```python
from build123d import *

# Parameters (mm, degrees)
SKETCH1_W           = 55
SKETCH1_H           = 4
SKETCH1_W_2         = 4.6
SKETCH1_H_2         = 5
BOSS_EXTRUDE2_DEPTH = 30
FILLET1_R           = 1
SKETCH2_R           = 2.5
SKETCH2_W           = 6.2
SKETCH2_H           = 6.2
CUT_EXTRUDE1_DEPTH  = 10
SKETCH4_W           = 19.295263263
SKETCH4_H           = 1.550295644
SKETCH4_W_2         = 7.637827672
SKETCH4_H_2         = 1.509017847
SKETCH4_W_3         = 7.600819518
SKETCH4_H_3         = 1.495167717
CUT_EXTRUDE2_DEPTH  = 25


with BuildPart() as part:
    # Sketch1 → Boss-Extrude2 (new body)
    with BuildSketch(Plane.XY):
        Rectangle(SKETCH1_W, SKETCH1_H)
        with Locations((-12.8, -4.5)):
            Rectangle(SKETCH1_W_2, SKETCH1_H_2)
        with Locations((12.8, -4.5)):
            Rectangle(SKETCH1_W_2, SKETCH1_H_2)
    extrude(amount=BOSS_EXTRUDE2_DEPTH)

    # Fillet1
    fillet1_edges = [part.edges().sort_by_distance(p)[0] for p in [
        (0, 2, 30),
        (0, 2, 0),
        (15.1, -7, 15),
        (10.5, -7, 15),
        (-10.5, -7, 15),
        (-15.1, -7, 15),
        (-27.5, 2, 15),
        (27.5, 2, 15),
    ]]
    fillet(fillet1_edges, radius=FILLET1_R)

    # Sketch2 → Cut-Extrude1 (cut)
    with BuildSketch(Plane(origin=(0, 2, 0), x_dir=(1, 0, 0), z_dir=(0, 1, 0))):
        with Locations(Location((-7, -6, 0), (0, 0, 270))):
            Circle(SKETCH2_R)
        with Locations(Location((-7, -14.949297523, 0), (0, 0, 270))):
            Circle(SKETCH2_R)
        with Locations(Location((-7, -23.898595046, 0), (0, 0, 270))):
            Circle(SKETCH2_R)
        with Locations(Location((7, -20, 0), (0, 0, 270))):
            Circle(SKETCH2_R)
        with Locations(Location((7, -10, 0), (0, 0, 270))):
            Circle(SKETCH2_R)
        with Locations((-20.5, -15)):
            Rectangle(SKETCH2_W, SKETCH2_H)
        with Locations((20.5, -15)):
            Rectangle(SKETCH2_W, SKETCH2_H)
    extrude(amount=-CUT_EXTRUDE1_DEPTH, mode=Mode.SUBTRACT)

    # Sketch4 → Cut-Extrude2 (cut)
    with BuildSketch(Plane.XY.offset(30)):
        with Locations((0.199720154, -1.224852178)):
            Rectangle(SKETCH4_W, SKETCH4_H)
        with Locations((-20.210751877, -1.245491077)):
            Rectangle(SKETCH4_W_2, SKETCH4_H_2)
        with Locations((20.547753604, -1.252416141)):
            Rectangle(SKETCH4_W_3, SKETCH4_H_3)
    extrude(amount=-CUT_EXTRUDE2_DEPTH, mode=Mode.SUBTRACT)


solid = part.part
```
Part model, mm, in its own coordinate system. A direction names the side the tool comes from. Round coordinates to 2 decimals unless told otherwise and drop trailing zeros. Order: outer loops, then holes, each group sorted by start corner. A loop starts at its lowest first (then second) coordinate and runs counter-clockwise, first axis right, second up. Notation, with made-up numbers: M 80,36 L 138,36 A23 cw 138,62 Z; hole C -26.5,84 d10. An arc over 180 degrees is marked long. Answer in a Markdown table with one row per item. Add a question column.
Q1. Cut at C-C on y = -4.5. Give the cut face in (x, z), and give its area (3 significant figures).
Q2. Mould opens along X. For faces 5 (the face through (-15.1, -4, 15)), 6 (the face through (0, -1, 0)), 7 (the face through (0, -0.45, 18)) say: +X half, -X half, draft (parallel to the pull), parting line (faces both ways), or undercut.
Q3. Wall check: L1, parallel to Z at x = -7, y = -0.4; L2, parallel to X at y = -0.65, z = 6; L3, parallel to X at y = 1.15, z = 10. Give the ranges that are in metal, low to high. Write a range as from..to.
Q4. Cut at D-D on x = 18.5. Give the cut face in (y, z).
Q5. 3-axis set-ups, long thin cutter, end or side, ignore diameter. For faces 1 (the face through (10.5, -4, 15)), 2 (the face through (-21, 1, 18.1)), 3 (the face through (25, -2, 11)), 4 (the face through (-20, -0.491, 20)): which of +Z, -Z, +X, -X, +Y, -Y reach the whole face in a straight line?
Q6. Cut at B-B on x = 7. Give the cut face in (y, z).
Q7. Pin check, flat tips, straight feed: pin 1 (1 mm diameter, centred on x = -4, z = 4, fed in from -Y); pin 2 (6 mm diameter, centred on x = 8, z = 25.5, fed in from -Y); pin 3 (15.5 mm diameter, centred on x = 3, z = 23.5, fed in from -Y); pin 4 (4 mm diameter, centred on x = -7, z = 14.95, fed in from +Y). Stop position of each tip, or through.
Established:
| question | item | result |
|---|---|---|
| 1 | outline | M -15.1,0 L -10.5,0 L -10.5,30 L -15.1,30 Z; M 10.5,0 L 15.1,0 L 15.1,30 L 10.5,30 Z |
| 1 | area | 276 mm2 |
| 2 | face 5 | -X half |
| 2 | face 6 | draft |
| 2 | face 7 | undercut |
| 3 | L1 | z = 0..3.5, 8.5..12.45, 17.45..21.4, 26.4..30 |
| 3 | L2 | x = -27.5..-24.03, -16.39..-9.5, 9.85..16.75, 24.35..27.5 |
| 3 | L3 | x = -27.49..4.5, 9.5..27.49 |
| 4 | outline | M -2,0 L 1,0 A1 ccw 2,1 L 2,11.9 L -0.5,11.9 L -0.5,5 L -2,5 Z; M -0.5,18.1 L 2,18.1 L 2,29 A1 ccw 1,30 L -0.5,30 Z |
| 5 | face 1 | +Z, -Z, -Y |
| 5 | face 2 | +Y, -Y |
| 5 | face 3 | +Z, -Z, +X, -Y |
| 5 | face 4 | +Z, -Y |
| 6 | outline | M -2,0 L 1,0 A1 ccw 2,1 L 2,7.5 L -0.45,7.5 L -0.45,5 L -2,5 Z; M -0.45,12.5 L 2,12.5 L 2,17.5 L -0.45,17.5 Z; M -0.45,22.5 L 2,22.5 L 2,29 A1 ccw 1,30 L -0.45,30 Z |
| 7 | pin 1 | stops at y = -2 |
| 7 | pin 2 | stops at y = -6.87 |
| 7 | pin 3 | stops at y = -6.66 |
| 7 | pin 4 | passes through |
